Read the model definition and answer for the solid it produces. Units are mm, in the model's axes. Face numbers are marked on the shaded views. A direction names the side the tool comes from. Coordinates: 2 decimals unless noted, no trailing zeros. Loops run counter-clockwise (first coordinate to the right, second up) from the corner with the lowest first, then second, coordinate; pieces in that order, holes last. Notation, with made-up numbers: (85, 66) - (134, 66) arc R14 ccw to (134, 84) - close; hole circle Ø6 at (-10, 45.25). An arc over 180 degrees is marked (long way). Use one line per item in the form item = value.
from build123d import *

# Parameters (mm, degrees)
SKETCH1_W               = 200
SKETCH1_H               = 200
BOSS_EXTRUDE1_DEPTH     = 50
CUT_EXTRUDE1_DEPTH      = 151
CUT_EXTRUDE1_DEPTH_BACK = 40
SKETCH2_W               = 180
SKETCH2_H               = 180
SKETCH3_W               = 21
SKETCH3_H               = 40
CUT_EXTRUDE2_DEPTH      = 40


with BuildPart() as part:
    # Sketch1 → Boss-Extrude1 (new body)
    with BuildSketch(Plane(origin=(0, 0, 0), x_dir=(1, 0, 0), z_dir=(0, 1, 0))):
        Rectangle(SKETCH1_W, SKETCH1_H)
    extrude(amount=BOSS_EXTRUDE1_DEPTH)

    # Sketch2 → Cut-Extrude1 (cut, two sides: drawn at the far end of the back side and taken through both)
    with BuildSketch(Plane(origin=(0, 50, 0), x_dir=(1, 0, 0), z_dir=(0, 1, 0)).offset(-CUT_EXTRUDE1_DEPTH_BACK)):
        Rectangle(SKETCH2_W, SKETCH2_H)
    extrude(amount=CUT_EXTRUDE1_DEPTH + CUT_EXTRUDE1_DEPTH_BACK, mode=Mode.SUBTRACT)

    # Sketch3 → Cut-Extrude2 (cut)
    with BuildSketch(Plane.XY.offset(100)):
        with Locations((0, 30)):
            Rectangle(SKETCH3_W, SKETCH3_H)
    extrude(amount=-CUT_EXTRUDE2_DEPTH, mode=Mode.SUBTRACT)


solid = part.part
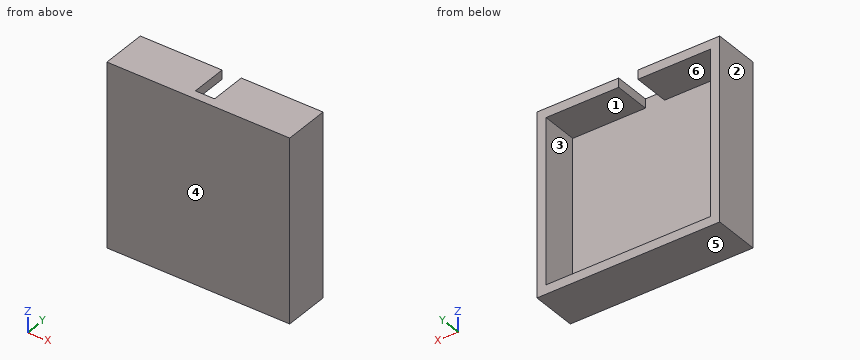
Item 1: Find the intervals of material crossed by L1, parallel to X at y = 28.5, z = 49; L2, parallel to Y at x = -82, z = 64, in increasing order.
Results below:
L1 = -100 to -90, 90 to 100
L2 = 0 to 10
Item 2: The part is cut by section C-C on y = 21.5. Give the vertices of the cut face in (x, z), plus the area to 3 significant figures.
Results below:
outline = (-100, -100) - (100, -100) - (100, 100) - (10.5, 100) - (10.5, 90) - (90, 90) - (90, -90) - (-90, -90) - (-90, 90) - (-10.5, 90) - (-10.5, 100) - (-100, 100) - close
area = 7,390 mm²
Item 3: The part is cut by section A-A on x = 51. Give the vertices of the cut face in (y, z), plus the area to 3 significant figures.
Results below:
outline = (0, -100) - (50, -100) - (50, -90) - (10, -90) - (10, 90) - (50, 90) - (50, 100) - (0, 100) - close
area = 2,800 mm²
Item 4: The part is cut by section D-D on x = -7. Give the vertices of the cut face in (y, z), plus the area to 3 significant figures.
Results below:
outline = (0, -100) - (50, -100) - (50, -90) - (10, -90) - (10, 100) - (0, 100) - close
area = 2,400 mm²
Item 5: For a pull along Z with two mould halves and no side action, classify the marked faces 3, 4, 5 and 6 as +Z half, -Z half, draft (parallel to the pull), parting line (faces both ways), or undercut.
Results below:
face_3 = undercut
face_4 = draft
face_5 = -Z half
face_6 = undercut
Item 6: The part is cut by section B-B on z = -42.5. Give the vertices of the cut face in (x, y), plus the area to 3 significant figures.
Results below:
outline = (-100, 0) - (100, 0) - (100, 50) - (90, 50) - (90, 10) - (-90, 10) - (-90, 50) - (-100, 50) - close
area = 2,800 mm²
Item 7: Which of the six approach directions +Z, -Z, +X, -X, +Y, -Y give full straight-line access (tool end or side, diameter ignored) to the marked faces 1 and 2?
Results below:
face_1 = +Y
face_2 = +Z, -Z, -X, +Y, -Y
Item 8: This flat-tipped pin is pushed along its axis until it touches: P1, Ø6, axis at x = 15, z = -59, coming from the +Y side. Where does it stop, or does it pass through?
Results below:
P1 = 10
